from build123d import *

# Parameters (mm, degrees)
SKETCH_1_W          = 56.451666402
SKETCH_1_H          = 55.81933344
SKETCH_1_R          = 6.008227446
EXTRUDE_1_DEPTH     = 6
SKETCH_2_R          = 5.984064553
EXTRUDE_2_DEPTH     = 32
SKETCH_3_R          = 8.240525962
EXTRUDE_3_DEPTH     = 32
SKETCH_2_3_R        = 5.984064553
CUT_EXTRUDE_2_DEPTH = 51.986735101


with BuildPart() as part:
    # Sketch 1 → Extrude 1 (new body)
    with BuildSketch(Plane.XY):
        Rectangle(SKETCH_1_W, SKETCH_1_H)
        with Locations((0, 15.26895552)):
            Circle(SKETCH_1_R, mode=Mode.SUBTRACT)
    extrude(amount=EXTRUDE_1_DEPTH)



with BuildPart() as body_2:
    # Sketch 2 → Extrude 2 (new body)
    with BuildSketch(Plane.XY.offset(6)):
        with Locations((-0.012037356, 15.289906593)):
            Circle(SKETCH_2_R)
    extrude(amount=EXTRUDE_2_DEPTH)


with BuildPart() as part_1:
    add(part.part)

    add(body_2.part)  # Extrude 3 merges body 2
    # Sketch 3 → Extrude 3 (add)
    with BuildSketch(Plane.XY.offset(6)):
        with Locations(Location((-0.006651179, 15.303273522, 0), (0, 0, 180))):
            Circle(SKETCH_3_R)
    extrude(amount=EXTRUDE_3_DEPTH)

    # Sketch 2_3 → Cut-Extrude 2 (cut, through all)
    with BuildSketch(Plane.XY.offset(6)):
        with Locations(Location((-0.012037356, 15.289906593, 0), (0, 0, 119.879351389))):
            Circle(SKETCH_2_3_R)
    extrude(amount=CUT_EXTRUDE_2_DEPTH, mode=Mode.SUBTRACT)


solid = part_1.part
Geometry: final body of the model. Coordinates: model frame, mm. Round coordinates to 2 decimals unless told otherwise and drop trailing zeros. Loops run counter-clockwise (first coordinate to the right, second up) from the corner with the lowest first, then second, coordinate; pieces in that order, holes last. Notation, with made-up numbers: (9, 47) - (30, 47) arc R27 cw to (30, 81) - close; hole circle Ø6 at (29, 31.5). An arc over 180 degrees is marked (long way). Write each question's results on one line, items separated by ' | '. Start each with the question number.
1) Cut plane C-C on z = 10.5. Return loops of the section in (x, y), then the cut area to 3 significant figures.
2) Line query: probe 1 along Y at (x, z) = (0, 2.85); probe 2 along Y at (x, z) = (-2.5, 11); probe 3 along Z at (x, y) = (11.5, 19). Output: solid intervals per line, ascending. Write a range as [from, to].
3) First-contact query: P1, Ø2, axis at x = -17.5, y = 3, coming from the +Z side; P2, Ø1, axis at x = -1.5, z = 7, coming from the +Y side. Flat tips, straight axial feed; report the tip coordinate or a pass-through.
4) Cut plane D-D on y = -12. Return loops of the section in (x, z), then the cut area to 3 significant figures.
5) Mould query, pull axis Y, two halves, no side actions, for faces 1 (the face through (-28.226, 0, 3)), 2 (the face through (-0.779, 21.225, 21.776)), 3 (the face through (1.78, 23.348, 21.776)). Classes: released by +Y, released by -Y, zero draft, split by the parting line, or undercut.
Verdict:
1) outline: circle Ø16.48 at (-0.01, 15.3); hole circle Ø11.97 at (-0.01, 15.29) | area: 101 mm2
2) probe 1: y = [-27.91, 9.26], [21.28, 27.91] | probe 2: y = [7.45, 9.85], [20.73, 23.16] | probe 3: z = [0, 6]
3) P1: stops at z = 6 | P2: stops at y = 23.48
4) outline: (-28.23, 0) - (28.23, 0) - (28.23, 6) - (-28.23, 6) - close | area: 339 mm2
5) face 1: zero draft | face 2: undercut | face 3: split by the parting line
